```python
from build123d import *

# Parameters (mm, degrees)
F0_W     = 255
F0_H     = 155
F0_R     = 19
F1_DEPTH = 95
F2_R     = 19
F2_W     = 50
F2_H     = 105
F2_W_2   = 127
F2_H_2   = 25
F3_DEPTH = 28
F4_W     = 41.4112506824
F4_H     = 105
F4_W_2   = 28
F5_DEPTH = 255.001


with BuildPart() as f1:
    # F0 (on Front) → F1 (new body)
    with BuildSketch(Plane.XZ):
        with Locations((127.5, 77.5)):
            Rectangle(F0_W, F0_H)
        with Locations((64, 77)):
            Circle(F0_R, mode=Mode.SUBTRACT)
        with Locations((191, 77)):
            Circle(F0_R, mode=Mode.SUBTRACT)
    extrude(amount=F1_DEPTH)

    # F2 (on face) → F3 (cut)
    with BuildSketch(Plane.XZ.offset(95)):
        Polygon((128, 130), (0, 130), (0, 25), (255, 25), (255, 130), align=None)
        with Locations((64, 77)):
            Circle(F2_R, mode=Mode.SUBTRACT)
        with Locations((191, 77)):
            Circle(F2_R, mode=Mode.SUBTRACT)
        with Locations((-25, 77.5)):
            Rectangle(F2_W, F2_H)
        with Locations((280, 77.5)):
            Rectangle(F2_W, F2_H)
        Polygon((255, 155), (255, 130), (305, 130), (305, 190.759062767), (128, 190.759062767), (128, 155), align=None)
        with Locations((191.5, 142.5)):
            Rectangle(F2_W_2, F2_H_2)
    extrude(amount=-F3_DEPTH, mode=Mode.SUBTRACT)

    # F4 (on face) → F5 (cut, through all)
    with BuildSketch(Plane.YZ.offset(255)):
        with Locations((20.7056253412, 77.5)):
            Rectangle(F4_W, F4_H)
        with Locations((-14, 77.5)):
            Rectangle(F4_W_2, F4_H)
    extrude(amount=-F5_DEPTH, mode=Mode.SUBTRACT)


solid = f1.part
```
Build history of the part. All positions in model axes, mm. A direction names the side the tool comes from. Give positions to 0.01 mm unless a question says otherwise; leave off trailing zeros. Loops run counter-clockwise (first coordinate to the right, second up) from the corner with the lowest first, then second, coordinate; pieces in that order, holes last.
Item 1: Slice it at D-D, the plane y = -48. List the corners of the cut face in (x, z).
Answers follow:
outline: (0, 0) - (255, 0) - (255, 155) - (0, 155) - close; hole circle Ø38 at (64, 77); hole circle Ø38 at (191, 77)
Item 2: Which spindle directions (+Z, -Z, +X, -X, +Y, -Y) get a long thin tool onto all of the face, cutting with end or side? Do faces 1 (the face through (126, -81, 25)), 2 (the face through (126, -36, 155)), 3 (the face through (129, -28, 77)). Say none if no direction does.
Answers follow:
face 1: +X, -X, -Y
face 2: +Z, +X, -X, +Y, -Y
face 3: +X, -X, +Y
Item 3: Slice it at B-B, the plane z = 77. List the corners of the cut face in (x, y), and give its area (3 significant figures).
Answers follow:
outline: (0, -67) - (45, -67) - (45, -28) - (0, -28) - close; (83, -67) - (172, -67) - (172, -28) - (83, -28) - close; (210, -67) - (255, -67) - (255, -28) - (210, -28) - close
area: 6,980 mm2
Item 4: Slice it at C-C, the plane y = -21. List the corners of the cut face in (x, z), and give its area (4 significant figures).
Answers follow:
outline: (0, 0) - (255, 0) - (255, 25) - (0, 25) - close; (0, 130) - (255, 130) - (255, 155) - (0, 155) - close
area: 12,750 mm2
Item 5: Slice it at A-A, the plane x = 64. List the corners of the cut face in (y, z), and give its area (3 significant figures).
Answers follow:
outline: (-95, 0) - (0, 0) - (0, 25) - (-28, 25) - (-28, 58) - (-67, 58) - (-67, 25) - (-95, 25) - close; (-95, 130) - (-67, 130) - (-67, 96) - (-28, 96) - (-28, 130) - (0, 130) - (0, 155) - (-95, 155) - close
area: 7,360 mm2
Item 6: Flat gauge pins, fed straight in: pin 1 (2 mm diameter, centred on x = 127, y = -68.5, fed in from -Z); pin 2 (8.5 mm diameter, centred on x = 149, y = -87, fed in from +Z); pin 3 (7.5 mm diameter, centred on y = -87.5, z = 147.5, fed in from +X); pin 4 (1.5 mm diameter, centred on x = 152, z = 95, fed in from +Y). Where does each tip first touch, or does it go through?
Answers follow:
pin 1: stops at z = 0
pin 2: stops at z = 25
pin 3: stops at x = 128
pin 4: stops at y = -28
Item 7: Pull direction X, two halves, no side cores. Call faces 4 (the face through (126, -67, 91)), 5 (the face through (188.53, -47.23, 95.84)), 6 (the face through (128, -81, 143)), 7 (the face through (61.53, -47.23, 95.84)): released by +X, released by -X, zero draft, split by the parting line, or undercut.
Answers follow:
face 4: zero draft
face 5: undercut
face 6: released by +X
face 7: undercut
Item 8: Drill centre lines: line 1 (X direction, y = -40, z = 77); line 2 (Z direction, x = 142, y = -14.5); line 3 (Z direction, x = 64, y = -37.5). Where is each one in solid material? Low to high.
Answers follow:
line 1: x = 0 to 45, 83 to 172, 210 to 255
line 2: z = 0 to 25, 130 to 155
line 3: z = 0 to 58, 96 to 155
